Check sheet for the modelled part. Datum: model origin and axes. Units: mm. Coordinates: 2 decimals unless noted, no trailing zeros. Loops run counter-clockwise (first coordinate to the right, second up) from the corner with the lowest first, then second, coordinate; pieces in that order, holes last.
from build123d import *

# Parameters (mm, degrees)
SKETCH_1_W          = 82
SKETCH_1_H          = 30
SKETCH_1_R          = 1.5
SKETCH_1_W_2        = 20
SKETCH_1_H_2        = 2
EXTRUDE_1_DEPTH     = 2
SKETCH_4_R          = 0.75
CUT_EXTRUDE_1_DEPTH = 51.842895276
SKETCH_5_W          = 31
SKETCH_5_H          = 6.5
SKETCH_5_H_2        = 7.5
CUT_EXTRUDE_2_DEPTH = 51.842895276
FILLET_1_R          = 1


with BuildPart() as part:
    # 草图1 → 凸台-拉伸1 (new body)
    with BuildSketch(Plane(origin=(0, 0, 0), x_dir=(1, 0, 0), z_dir=(0, 1, 0))):
        with Locations((0, 15)):
            Rectangle(SKETCH_1_W, SKETCH_1_H)
        with Locations(Location((-37.5, 26, 0), (0, 0, 270))):
            Circle(SKETCH_1_R, mode=Mode.SUBTRACT)
        with Locations(Location((-37.5, 4, 0), (0, 0, 270))):
            Circle(SKETCH_1_R, mode=Mode.SUBTRACT)
        with Locations(Location((37.5, 26, 0), (0, 0, 270))):
            Circle(SKETCH_1_R, mode=Mode.SUBTRACT)
        with Locations(Location((37.5, 4, 0), (0, 0, 270))):
            Circle(SKETCH_1_R, mode=Mode.SUBTRACT)
        with Locations((17, 14.5)):
            Rectangle(SKETCH_1_W_2, SKETCH_1_H_2, mode=Mode.SUBTRACT)
        with Locations((-18, 14.5)):
            Rectangle(SKETCH_1_W_2, SKETCH_1_H_2, mode=Mode.SUBTRACT)
    extrude(amount=EXTRUDE_1_DEPTH)

    # 草图4 → 切除-拉伸1 (cut, through all)
    with BuildSketch(Plane(origin=(0, 2, 0), x_dir=(1, 0, 0), z_dir=(0, 1, 0))):
        with Locations((-27.25, 15.5)):
            Circle(SKETCH_4_R)
        with Locations((-27.25, 13.5)):
            Circle(SKETCH_4_R)
        with Locations((-8.75, 15.5)):
            Circle(SKETCH_4_R)
        with Locations((-8.75, 13.5)):
            Circle(SKETCH_4_R)
        with Locations((7.75, 15.5)):
            Circle(SKETCH_4_R)
        with Locations((7.75, 13.5)):
            Circle(SKETCH_4_R)
        with Locations((26.25, 15.5)):
            Circle(SKETCH_4_R)
        with Locations((26.25, 13.5)):
            Circle(SKETCH_4_R)
    extrude(amount=-CUT_EXTRUDE_1_DEPTH, mode=Mode.SUBTRACT)

    # 草图5 → 切除-拉伸2 (cut, through all)
    with BuildSketch(Plane(origin=(0, 2, 0), x_dir=(1, 0, 0), z_dir=(0, 1, 0))):
        with Locations((-18, 7.25)):
            Rectangle(SKETCH_5_W, SKETCH_5_H)
        with Locations((-18, 22.25)):
            Rectangle(SKETCH_5_W, SKETCH_5_H_2)
        with Locations((17, 22.25)):
            Rectangle(SKETCH_5_W, SKETCH_5_H_2)
        with Locations((17, 7.25)):
            Rectangle(SKETCH_5_W, SKETCH_5_H)
    extrude(amount=-CUT_EXTRUDE_2_DEPTH, mode=Mode.SUBTRACT)

    # 圆角1
    fillet_1_edges = [part.edges().sort_by_distance(p)[0] for p in [
        (1.5, 1, -10.5),
        (32.5, 1, -10.5),
        (32.5, 1, -4),
        (1.5, 1, -4),
        (1.5, 1, -26),
        (32.5, 1, -26),
        (32.5, 1, -18.5),
        (1.5, 1, -18.5),
        (-33.5, 1, -18.5),
        (-33.5, 1, -26),
        (-2.5, 1, -26),
        (-2.5, 1, -18.5),
        (-33.5, 1, -4),
        (-33.5, 1, -10.5),
        (-2.5, 1, -10.5),
        (-2.5, 1, -4),
        (-41, 1, -30),
        (41, 1, -30),
        (41, 1, 0),
        (-41, 1, 0),
    ]]
    fillet(fillet_1_edges, radius=FILLET_1_R)


solid = part.part
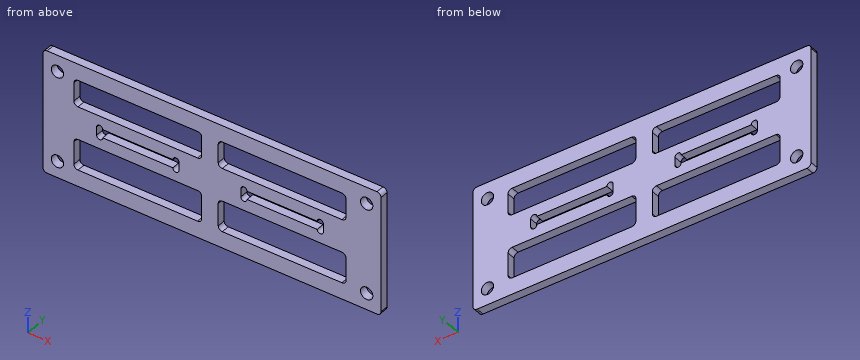
(1) Section check D-D, the plane y = 0.45. Count the separate pieces of the cut face and the enclosed holes in it, plus the area to 3 significant figures.
(2) Section check B-B, the plane x = -5. Enter the section's corners in (y, z).
(3) Scan lines: line 1 along X through (y, z) = (0.3, -21.75); line 2 along Z through (x, y) = (-30, 0.75); line 3 along Z through (x, y) = (-11, 1). Record each from-to range of solid material in increasing order.
(4) Gauge pin test, flat ends, axial feed: P1, Ø2.5, axis at x = -37.5, z = -26, coming from the +Y side; P2, Ø8, axis at x = -30, z = -22.5, coming from the +Y side. Record the tip position at first contact, or that the pin passes through.
(5) Section check A-A, the plane x = -25. Enter the section's corners in (y, z).
(6) Section check C-C, the plane z = -6.25. Enter the section's corners in (x, y), plus the area to 3 significant figures.
Determined:
1. separate pieces: 1
1. enclosed holes: 10
1. area: 1,480 mm2
2. outline: (0, -30) - (2, -30) - (2, -26) - (0, -26) - close; (0, -18.5) - (2, -18.5) - (2, -10.5) - (0, -10.5) - close; (0, -4) - (2, -4) - (2, 0) - (0, 0) - close
3. line 1: x = -41 to -33.5, -2.5 to 1.5, 32.5 to 41
3. line 2: z = -30 to -26, -18.5 to -10.5, -4 to 0
3. line 3: z = -30 to -26, -18.5 to -15.5, -13.5 to -10.5, -4 to 0
4. P1: passes through
4. P2: stops at y = 2
5. outline: (0, -30) - (2, -30) - (2, -26) - (0, -26) - close; (0, -18.5) - (2, -18.5) - (2, -15.5) - (0, -15.5) - close; (0, -13.5) - (2, -13.5) - (2, -10.5) - (0, -10.5) - close; (0, -4) - (2, -4) - (2, 0) - (0, 0) - close
6. outline: (-41, 0) - (-33.5, 0) - (-33.5, 2) - (-41, 2) - close; (-2.5, 0) - (1.5, 0) - (1.5, 2) - (-2.5, 2) - close; (32.5, 0) - (41, 0) - (41, 2) - (32.5, 2) - close
6. area: 40.0 mm2
